Could you check a few things on this model? Use its own coordinates, in mm. A direction names the side the tool comes from. Coordinates: 2 decimals unless noted, no trailing zeros. Order: outer loops, then holes, each group sorted by start corner. A loop starts at its lowest first (then second) coordinate and runs counter-clockwise, first axis right, second up. Notation, with made-up numbers: (43, -21.5) -> (77, -21.5) arc R21 ccw to (77, 6.5) -> close; hole circle Ø5 at (53, 12). An arc over 180 degrees is marked (long way). Put each result on its own line as item: value. Start each with the question number.
Q1. If we section it at C-C (x = 8): Please give me the cut outline in (y, z), and give its area (3 significant figures).
Q2. Please list where these lines run through material, in increasing order: line 1 along X through (y, z) = (0.55, 476.25); line 2 along X through (y, z) = (44, 215); line 3 along Y through (x, z) = (5.5, 366.5).
Q3. If we section it at B-B (z = 462): Please give me the cut outline in (x, y).
Q4. If we section it at A-A (y = 22.5): Please give me the cut outline in (x, z).
Q5. Will these pins go through, and if not, where does the flat tip stop? pin 1 (4 mm diameter, centred on y = 30, z = 197, fed in from -X); pin 2 (15 mm diameter, centred on x = 16, z = 321.5, fed in from +Y).
Q6. For faces 4 (the face through (49.212, 27, 263)), 5 (the face through (18.91, 0.78, 54.65)), which set-ups out of +Z, -Z, +X, -X, +Y, -Y let a thin tool reach every point of the face, with its end or its side?
Q7. We'd pull the mould along X, two halves only. Please class faces 1 (the face through (19.138, 0.783, 21.822)), 2 (the face through (50.8, 25, 263)), 3 (the face through (25, 0, 263)): +X half, -X half, draft (parallel to the pull), parting line (faces both ways), or undercut.
from build123d import *

# Parameters (mm, degrees)
EXTRUDE1_DEPTH     = 533.4
SKETCH2_R          = 4.1021
CUT_EXTRUDE1_DEPTH = 51.8


with BuildPart() as part:
    # Sketch1 → Extrude1 (new body)
    with BuildSketch(Plane.XY):
        Polygon((0, 0), (50.8, 0), (50.8, 50.8), (49.2125, 50.8), (49.2125, 1.5875), (0, 1.5875), align=None)
    extrude(amount=EXTRUDE1_DEPTH)

    # Sketch2 → Cut-Extrude1 (cut, through all)
    with BuildSketch(Plane.XZ):
        with Locations((22.1615, 57.15)):
            Circle(SKETCH2_R)
        with Locations((22.1615, 476.25)):
            Circle(SKETCH2_R)
        with Locations((22.1615, 19.05)):
            Circle(SKETCH2_R)
        with BuildLine():
            Line((22.1615, 518.4521), (34.8615, 518.4521))
            ThreePointArc((34.8615, 518.4521), (38.9636, 514.35), (34.8615, 510.2479))
            Line((34.8615, 510.2479), (22.1615, 510.2479))
            ThreePointArc((22.1615, 510.2479), (18.0594, 514.35), (22.1615, 518.4521))
        make_face()
    extrude(amount=-CUT_EXTRUDE1_DEPTH, mode=Mode.SUBTRACT)


solid = part.part
The answers:
1. outline: (0, 0) -> (1.59, 0) -> (1.59, 533.4) -> (0, 533.4) -> close
1. area: 847 mm^2
2. line 1: 0 to 18.06, 26.26 to 50.8
2. line 2: 49.21 to 50.8
2. line 3: 0 to 1.59
3. outline: (0, 0) -> (50.8, 0) -> (50.8, 50.8) -> (49.21, 50.8) -> (49.21, 1.59) -> (0, 1.59) -> close
4. outline: (49.21, 0) -> (50.8, 0) -> (50.8, 533.4) -> (49.21, 533.4) -> close
5. pin 1: x = 49.21
5. pin 2: y = 1.59
6. face 4: +Z, -Z, -X, +Y
6. face 5: +Y, -Y
7. face 1: undercut
7. face 2: +X half
7. face 3: draft
